from build123d import *

# Parameters (mm, degrees)
F0_W     = 77
F0_H     = 60
F1_DEPTH = 3.5
F3_DEPTH = 3.5
F5_DEPTH = 3.5


with BuildPart() as f1:
    # F0 (on Top) → F1 (new body)
    with BuildSketch(Plane.XY):
        Rectangle(F0_W, F0_H)
    extrude(amount=F1_DEPTH)

    # F2 (on face) → F3 (cut)
    with BuildSketch(Plane(origin=(-38.5, 0, 0), x_dir=(0, -1, 0), z_dir=(-1, 0, 0))):
        Polygon((-16, 3.5), (-30, 3.5), (-30, 0), (-18, 0), align=None)
        Polygon((10, 3.5), (-10, 3.5), (-8, 0), (8, 0), align=None)
        Polygon((30, 3.5), (16, 3.5), (18, 0), (30, 0), align=None)
    extrude(amount=-F3_DEPTH, mode=Mode.SUBTRACT)

    # F4 (on face) → F5 (cut)
    with BuildSketch(Plane.YZ.offset(38.5)):
        Polygon((-18, 0), (-16, 3.5), (-30, 3.5), (-30, 0), align=None)
        Polygon((8, 0), (10, 3.5), (-10, 3.5), (-8, 0), align=None)
        Polygon((30, 0), (30, 3.5), (16, 3.5), (18, 0), align=None)
    extrude(amount=-F5_DEPTH, mode=Mode.SUBTRACT)


solid = f1.part
Can you work these out from the model? Positions are in its coordinate system, mm. A direction names the side the tool comes from. Round coordinates to 2 decimals unless told otherwise and drop trailing zeros. Write each loop counter-clockwise with the first axis right and the second up, starting at its lowest first coordinate (ties: lowest second). Pieces come first, ordered by that corner, then holes. Notation, with made-up numbers: M -18.5,67.25 L 16.5,67.25 A30 ccw 16.5,93.25 Z; hole C 56.5,88 d4. An arc over 180 degrees is marked long. Use a Markdown table: item, result.
Item 1: I want a section at C-C (y = 3). List the corners of the cut face in (x, z) for me, and give its area (3 significant figures).
Found:
| item | result |
|---|---|
| outline | M -35,0 L 35,0 L 35,3.5 L -35,3.5 Z |
| area | 245 mm2 |
Item 2: I want a section at B-B (z = 1.85). List the corners of the cut face in (x, y) for me.
Found:
| item | result |
|---|---|
| outline | M -38.5,-16.94 L -35,-16.94 L -35,-30 L 35,-30 L 35,-16.94 L 38.5,-16.94 L 38.5,-9.06 L 35,-9.06 L 35,9.06 L 38.5,9.06 L 38.5,16.94 L 35,16.94 L 35,30 L -35,30 L -35,16.94 L -38.5,16.94 L -38.5,9.06 L -35,9.06 L -35,-9.06 L -38.5,-9.06 Z |
Item 3: Which directions (+Z, -Z, +X, -X, +Y, -Y) give clear straight access to the entire face, cutting with the end or side of a thin tool? Please do faces 5 (the face through (-36.77, -16.99, 1.77)), 6 (the face through (36.77, 16.99, 1.77)), 7 (the face through (-36.77, 9.01, 1.77)), 8 (the face through (-36.77, 17.01, 1.73)).
Found:
| item | result |
|---|---|
| face 5 | +Z, -X, -Y |
| face 6 | +Z, +X, +Y |
| face 7 | +Z, -X |
| face 8 | +Z, -X, +Y |
Item 4: I want a section at A-A (y = -17). List the corners of the cut face in (x, z) for me, and give its area (3 significant figures).
Found:
| item | result |
|---|---|
| outline | M -38.5,0 L 38.5,0 L 38.5,1.75 L 35,1.75 L 35,3.5 L -35,3.5 L -35,1.75 L -38.5,1.75 Z |
| area | 257 mm2 |
Item 5: If I drill on line 1 along X through (y, z) = (-20, 2.35); line 2 along Y through (x, z) = (35.5, 0.9), over which ranges is the centre line in solid material (lowest first)? Write a range as [from, to].
Found:
| item | result |
|---|---|
| line 1 | x = [-35, 35] |
| line 2 | y = [-17.49, -8.51], [8.51, 17.49] |
Item 6: For pin 1 Ø1.8 at (y, z) = (25.5, 2) entering from +X; pin 2 Ø1.8 at (y, z) = (-4.5, 2) entering from -X, each with a flat end and sliding along its axis, tell me the tip position at first contact or that it passes through.
Found:
| item | result |
|---|---|
| pin 1 | stops at x = 35 |
| pin 2 | stops at x = -35 |
Item 7: We'd pull the mould along Y, two halves only. Please class faces 1 (the face through (-1, 0, 3.5)), 2 (the face through (36.77, -17.01, 1.73)), 3 (the face through (36.77, 8.99, 1.73)), 4 (the face through (0, 30, 2)): released by +Y, released by -Y, zero draft, split by the parting line, or undercut.
Found:
| item | result |
|---|---|
| face 1 | zero draft |
| face 2 | released by -Y |
| face 3 | undercut |
| face 4 | released by +Y |
